Input: part model. Units: mm. Frame: model coordinates. A direction names the side the tool comes from. Coordinates: 2 decimals unless noted, no trailing zeros. Loops run counter-clockwise (first coordinate to the right, second up) from the corner with the lowest first, then second, coordinate; pieces in that order, holes last.
(1) Set-up query: faces 1 (the face through (6, 13, -580.8)), 2 (the face through (-6, 13, 579.6)), 3 (the face through (-431, 25.4, 48)). Return all of +Z, -Z, +X, -X, +Y, -Y with unobstructed straight access to the full face (end or side cutting, diameter ignored); none if empty.
(2) Line query: L1, parallel to Z at x = 7.5, y = 18; L2, parallel to X at y = 22.75, z = 4.5. Output: solid intervals per line, ascending.
(3) Section B-B, the plane x = 155. Return loops of the section in (y, z).
(4) Mould query, pull axis X, two halves, no side actions, for faces 4 (the face through (-448.8, 13, -8)), 5 (the face through (-6, 13, 605)). Classes: released by +X, released by -X, zero draft, split by the parting line, or undercut.
(5) Section A-A, the plane z = -462. Return loops of the section in (x, y).
```python
from build123d import *

# Parameters (mm, degrees)
SKETCH2_W   = 25.4
SKETCH2_H   = 25.4
SKETCH2_W_2 = 23
SKETCH2_H_2 = 23


with BuildPart() as part:
    # Sweep1: sweep along a path in Sketch1
    with BuildLine(Plane(origin=(0, 0, 0), x_dir=(1, 0, 0), z_dir=(0, 1, 0))) as sweep1_path:
        Line((-450, 605), (450, 605))
        Line((450, 605), (450, -605))
        Line((450, -605), (-450, -605))
        Line((-450, -605), (-450, 605))
    # Sketch2 → Sweep1 (sweep)
    with BuildSketch(Plane(origin=(0, 0, 0), x_dir=(0, 0, -1), z_dir=(1, 0, 0))):
        with Locations((-592.3, 12.7)):
            Rectangle(SKETCH2_W, SKETCH2_H)
        with Locations((-592.3, 12.7)):
            Rectangle(SKETCH2_W_2, SKETCH2_H_2, mode=Mode.SUBTRACT)
    sweep(path=sweep1_path.line, transition=Transition.RIGHT)


solid = part.part
```
Report:
1. face 1: none
1. face 2: +Y, -Y
1. face 3: +Z, -Z, +X, -X, +Y
2. L1: z = -605 to -603.8, -580.8 to -579.6, 579.6 to 580.8, 603.8 to 605
2. L2: x = -450 to -448.8, -425.8 to -424.6, 424.6 to 425.8, 448.8 to 450
3. outline: (0, -605) - (25.4, -605) - (25.4, -579.6) - (0, -579.6) - close; (0, 579.6) - (25.4, 579.6) - (25.4, 605) - (0, 605) - close; hole (1.2, -603.8) - (24.2, -603.8) - (24.2, -580.8) - (1.2, -580.8) - close; hole (1.2, 580.8) - (24.2, 580.8) - (24.2, 603.8) - (1.2, 603.8) - close
4. face 4: undercut
4. face 5: zero draft
5. outline: (-450, 0) - (-424.6, 0) - (-424.6, 25.4) - (-450, 25.4) - close; (424.6, 0) - (450, 0) - (450, 25.4) - (424.6, 25.4) - close; hole (-448.8, 1.2) - (-425.8, 1.2) - (-425.8, 24.2) - (-448.8, 24.2) - close; hole (425.8, 1.2) - (448.8, 1.2) - (448.8, 24.2) - (425.8, 24.2) - close
